from build123d import *

# Parameters (mm, degrees)
F0_R     = 9.5
F1_DEPTH = 20
F2_R     = 5
F3_DEPTH = 8
F4_R     = 0.5
F5_SIZE  = 1
F6_W     = 1
F6_H     = 2


with BuildPart() as f1:
    # F0 (on Top) → F1 (new body)
    with BuildSketch(Plane.XY):
        Circle(F0_R)
    extrude(amount=-F1_DEPTH)

    # F2 (on face) → F3 (join)
    with BuildSketch(Plane.XY):
        Circle(F2_R)
    extrude(amount=F3_DEPTH)

    # F4
    f4_edges = [f1.edges().sort_by_distance(p)[0] for p in [
        (-9.5, 0, -20),
        (-9.5, 0, 0),
    ]]
    fillet(f4_edges, radius=F4_R)

    # F5
    f5_edges = [f1.edges().sort_by_distance(p)[0] for p in [
        (-5, 0, 8),
    ]]
    chamfer(f5_edges, length=F5_SIZE)

    # F6 (on Right) → F7 (revolve, cut)
    with BuildSketch(Plane.YZ):
        with Locations((-4.5, 1)):
            Rectangle(F6_W, F6_H)
    revolve(axis=Axis((0, 0, 7.854766), (0, 0, 1)), mode=Mode.SUBTRACT)


solid = f1.part
CAD build for the part. Positions are in the model's coordinates, mm. A direction names the side the tool comes from. Round coordinates to 2 decimals unless told otherwise and drop trailing zeros. Write each loop counter-clockwise with the first axis right and the second up, starting at its lowest first coordinate (ties: lowest second). Pieces come first, ordered by that corner, then holes. Notation, with made-up numbers: M -36.5,4 L 2.5,4 A31 ccw 2.5,29 Z; hole C -32,16.25 d3. An arc over 180 degrees is marked long. Put each result on its own line as item: value. Start each with the question number.
1) 3-axis set-ups, long thin cutter, end or side, ignore diameter. For faces 4 (the cylindrical face through (4.77, 1.5, 4.46)), 5 (the flat face through (4, -2, 0)), 6 (the flat face through (0, 0, -20)): which of +Z, -Z, +X, -X, +Y, -Y reach the whole face in a straight line?
2) Saw through at D-D, the plane z = -14. Write the cut outline in (x, y), and give its area (3 significant figures).
3) Saw through at C-C, the plane z = 6.25. Write the cut outline in (x, y).
4) Pin check, flat tips, straight feed: pin 1 Ø3 at (x, y) = (5.5, -1) entering from +Z; pin 2 Ø2 at (x, z) = (2, -13.5) entering from -Y; pin 3 Ø5 at (x, z) = (-4, -8.5) entering from +Y. Stop position of each tip, or through.
5) Saw through at A-A, the plane y = 0. Write the cut outline in (x, z).
6) Drill centre lines: probe 1 along Z at (x, y) = (0, -4.5); probe 2 along X at (y, z) = (0.25, -2). Where is each one in solid material? Low to high. Write a range as [from, to].
7) Pull direction Z, two halves, no side cores. Call faces 1 (the flat face through (0, 0, 8)), 2 (the cylindrical face through (-3.905, 0.867, 1.014)), 3 (the cylindrical face through (4.38, -8.43, -9.87)): pulls with the +Z half, pulls with the -Z half, needs draft (parallel to the pull), parting line crosses it, or undercut.
Resolved:
1. face 4: +Z
1. face 5: none
1. face 6: -Z, +X, -X, +Y, -Y
2. outline: C 0,0 d19
2. area: 284 mm²
3. outline: C 0,0 d10
4. pin 1: z = 7.91
4. pin 2: y = -9.45
4. pin 3: y = 9.38
5. outline: M -9.5,-19.5 A0.5 ccw -9,-20 L 9,-20 A0.5 ccw 9.5,-19.5 L 9.5,-0.5 A0.5 ccw 9,0 L 4,0 L 4,2 L 5,2 L 5,7 L 4,8 L -4,8 L -5,7 L -5,2 L -4,2 L -4,0 L -9,0 A0.5 ccw -9.5,-0.5 Z
6. probe 1: [-20, 0], [2, 7.5]
6. probe 2: [-9.5, 9.5]
7. face 1: pulls with the +Z half
7. face 2: undercut
7. face 3: needs draft
